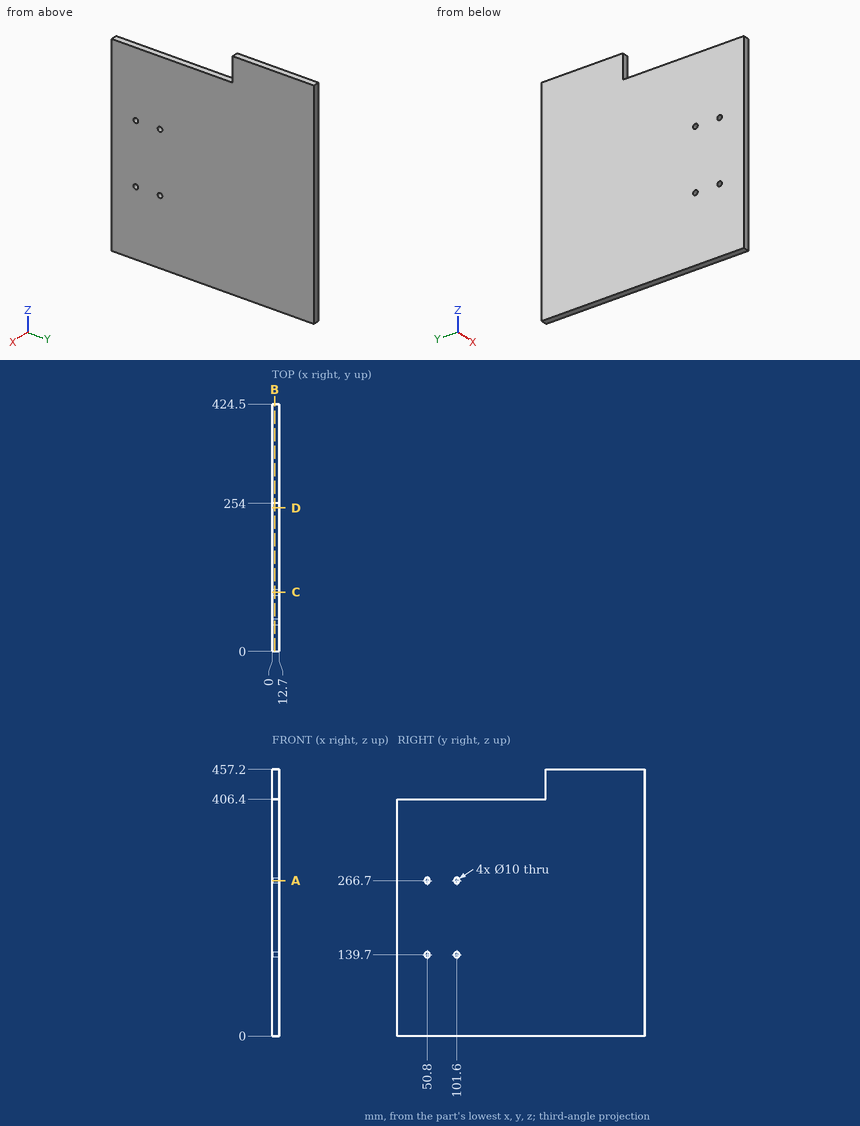
Print and shaded views of the part. All mm, measured from the part's lowest x, y and z. Give positions to 0.01 mm unless a question says otherwise; leave off trailing zeros. Write each loop counter-clockwise with the first axis right and the second up, starting at its lowest first coordinate (ties: lowest second). Pieces come first, ordered by that corner, then holes. Notation, with made-up numbers: (73.5, 3.25) - (116.5, 3.25) arc R21 ccw to (116.5, 9.25) - close; hole circle Ø5 at (44, 82.25). An arc over 180 degrees is marked (long way). One line per question, with ' | ' between items. Start each with the question number.
(1) Slice it at D-D on y = 246.5. Write the cut outline in (x, z).
(2) Wall check: line 1 along Y through (x, z) = (4.25, 266.7); line 2 along Z through (x, y) = (8.5, 94.5); line 3 along Y through (x, z) = (5.75, 422.5). Give the ranges that are in metal, low to high. Write a range as from..to.
(3) Slice it at A-A on z = 266.7. Write the cut outline in (x, y).
(4) Slice it at C-C on y = 101.6. Write the cut outline in (x, z).
(5) Slice it at B-B on x = 4.25. Write the cut outline in (y, z).
(6) Pin check, flat tips, straight feed: P1, Ø6, axis at x = 6, y = 145, coming from the -Z side; P2, Ø4, axis at x = 7, z = 420, coming from the -Y side. Stop position of each tip, or through.
Results below:
1) outline: (0, 0) - (12.7, 0) - (12.7, 406.4) - (0, 406.4) - close
2) line 1: 0..45.8, 55.8..96.6, 106.6..424.5 | line 2: 0..406.4 | line 3: 254..424.5
3) outline: (0, 0) - (12.7, 0) - (12.7, 45.8) - (0, 45.8) - close; (0, 55.8) - (12.7, 55.8) - (12.7, 96.6) - (0, 96.6) - close; (0, 106.6) - (12.7, 106.6) - (12.7, 424.5) - (0, 424.5) - close
4) outline: (0, 0) - (12.7, 0) - (12.7, 134.7) - (0, 134.7) - close; (0, 144.7) - (12.7, 144.7) - (12.7, 261.7) - (0, 261.7) - close; (0, 271.7) - (12.7, 271.7) - (12.7, 406.4) - (0, 406.4) - close
5) outline: (0, 0) - (424.5, 0) - (424.5, 457.2) - (254, 457.2) - (254, 406.4) - (0, 406.4) - close; hole circle Ø10 at (50.8, 139.7); hole circle Ø10 at (50.8, 266.7); hole circle Ø10 at (101.6, 139.7); hole circle Ø10 at (101.6, 266.7)
6) P1: z = 0 | P2: y = 254
